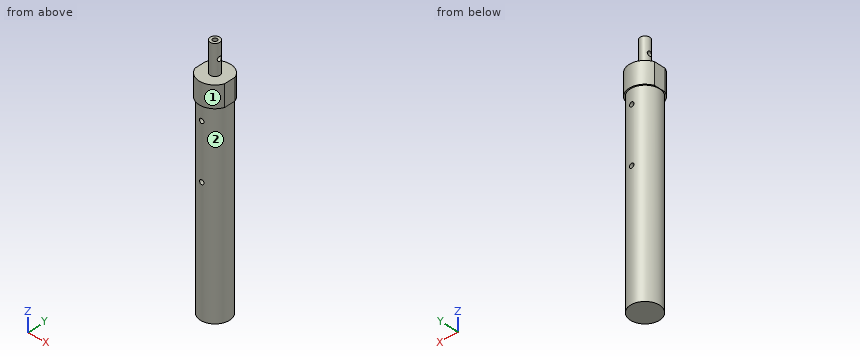
from build123d import *

# Parameters (mm, degrees)
SKETCH1_R                 = 8.73125
BOSS_EXTRUDE1_DEPTH       = 129.54
SKETCH2_R                 = 2.921
BOSS_EXTRUDE2_DEPTH       = 17.78
F_6_32_TAPPED_HOLE1_D     = 2.7051
F_6_32_TAPPED_HOLE2_D     = 2.7051
BOSS_EXTRUDE3_DEPTH       = 12.827
F_6_32_TAPPED_HOLE3_D     = 2.7051
F_6_32_TAPPED_HOLE3_DEPTH = 5.08
F_6_32_TAPPED_HOLE3_TIP   = 0.81269403


with BuildPart() as part:
    # Sketch1 → Boss-Extrude1 (new body)
    with BuildSketch(Plane.XY):
        Circle(SKETCH1_R)
    extrude(amount=BOSS_EXTRUDE1_DEPTH)

    # Sketch2 → Boss-Extrude2 (add)
    with BuildSketch(Plane.XY.offset(129.54)):
        Circle(SKETCH2_R)
    extrude(amount=BOSS_EXTRUDE2_DEPTH)

    # #6-32 Tapped Hole1 (through all)
    with Locations(Plane(origin=(0, 8.73125, 0), x_dir=(1, 0, 0), z_dir=(0, 1, 0))):
        with Locations((0, -74.93), (0, -107.95)):
            Hole(F_6_32_TAPPED_HOLE1_D / 2)

    # #6-32 Tapped Hole2 (through all)
    with Locations(Plane(origin=(2.921, 0, 0), x_dir=(0, 0, -1), z_dir=(1, 0, 0))):
        with Locations((-138.43, 0)):
            Hole(F_6_32_TAPPED_HOLE2_D / 2)

    # Sketch10 → Boss-Extrude3 (add)
    with BuildSketch(Plane.XY.offset(129.54)):
        with BuildLine():
            Line((8.89, -3.419579653), (8.89, 3.419579653))
            ThreePointArc((8.89, 3.419579653), (0, 9.525), (-8.89, 3.419579653))
            Line((-8.89, 3.419579653), (-8.89, -3.419579653))
            ThreePointArc((-8.89, -3.419579653), (0, -9.525), (8.89, -3.419579653))
        make_face()
    extrude(amount=-BOSS_EXTRUDE3_DEPTH)

    # #6-32 Tapped Hole3
    with Locations(Plane.XY.offset(147.32)):
        with Locations((0, 0)):
            Hole(F_6_32_TAPPED_HOLE3_D / 2, depth=F_6_32_TAPPED_HOLE3_DEPTH)
            with Locations((0, 0, -(F_6_32_TAPPED_HOLE3_DEPTH + F_6_32_TAPPED_HOLE3_TIP / 2))):  # 118° drill point
                Cone(0, F_6_32_TAPPED_HOLE3_D / 2, F_6_32_TAPPED_HOLE3_TIP, mode=Mode.SUBTRACT)


solid = part.part
Work out the finished part from the listing and answer in its coordinate system (mm). Face numbers are marked on the shaded views. A direction names the side the tool comes from. Give positions to 0.01 mm unless a question says otherwise; leave off trailing zeros. Order: outer loops, then holes, each group sorted by start corner. A loop starts at its lowest first (then second) coordinate and runs counter-clockwise, first axis right, second up. Notation, with made-up numbers: (80, 1.5) - (97, 1.5) arc R28 cw to (97, 35.5) - close; hole circle Ø8 at (84.5, 30). An arc over 180 degrees is marked (long way). Answer as CSV lines item,"result". Start each with the question number.
Q1. The part is cut by section D-D (z = 107.95). Write down the section's boundary in (x, y), then the cut area to 3 significant figures.
Q2. For the marked faces 1 and 2, determine the directions among +Z, -Z, +X, -X, +Y, -Y from which every point of the face is accessible in a straight line to the end or side of a thin tool.
Q3. Given pin 1 Ø2 at (y, z) = (0, 138.43) entering from -X; pin 2 Ø8 at (y, z) = (5, 103.5) entering from -X; pin 3 Ø9 at (x, y) = (3, 3.5) entering from +Z; pin 4 Ø1.5 at (x, z) = (7, 110) entering from +Y, each flat-ended and moving along its own axis, determine where each tip first touches the part or whether it passes through.
Q4. The part is cut by section B-B (x = -6.25). Write down the section's boundary in (y, z), then the cut area to 3 significant figures.
Q5. The part is cut by section A-A (y = 6). Write down the section's boundary in (x, z).
Q6. Find the intervals of material crossed by L1, parallel to Z at x = 0, y = -4.25; L2, parallel to Z at x = 1.1, y = 0; L3, parallel to Z at x = 5.25, y = 6.25, in increasing order. Write a range as [from, to].
Q7. The part is cut by section C-C (z = 21.5). Write down the section's boundary in (x, y).
Check result:
1,outline,"(-1.35, -8.63) - (-1.35, 8.63) arc R8.73 ccw to start; (1.35, -8.63) arc R8.73 ccw to (1.35, 8.63) - close"
1,area,"192 mm²"
2,face 1,"+Z, -Z, -Y"
2,face 2,"-Z"
3,pin 1,"passes through"
3,pin 2,"stops at x = -8.67"
3,pin 3,"stops at z = 147.32"
3,pin 4,"stops at y = 6.1"
4,outline,"(-7.19, 116.71) - (-6.1, 116.71) - (-6.1, 0) - (6.1, 0) - (6.1, 116.71) - (7.19, 116.71) - (7.19, 129.54) - (-7.19, 129.54) - close"
4,area,"1,610 mm²"
5,outline,"(-7.4, 116.71) - (-6.34, 116.71) - (-6.34, 0) - (6.34, 0) - (6.34, 116.71) - (7.4, 116.71) - (7.4, 129.54) - (-7.4, 129.54) - close; hole circle Ø2.71 at (0, 74.93); hole circle Ø2.71 at (0, 107.95)"
6,L1,"z = [0, 73.58], [76.28, 106.6], [109.3, 129.54]"
6,L2,"z = [0, 74.14], [75.72, 107.16], [108.74, 137.08], [139.78, 142.09]"
6,L3,"z = [0, 129.54]"
7,outline,"circle Ø17.46 at (0, 0)"
